from build123d import *

# Parameters (mm, degrees)
BOSS_EXTRUDE1_DEPTH = 13.85


with BuildPart() as part:
    # Sketch1 → Boss-Extrude1 (new, symmetric)
    with BuildSketch(Plane(origin=(0, 0, 0), x_dir=(0, 0, -1), z_dir=(1, 0, 0))):
        with BuildLine():
            ThreePointArc((75, 0), (-54.60082417, 51.417409503), (4.5, -74.864878281))
            Line((4.5, -74.864878281), (4.458, -74.166139417))
            ThreePointArc((4.458, -74.166139417), (-54.091216477, 50.937513681), (74.3, 0))
            ThreePointArc((74.3, 0), (66.712592514, -32.709631609), (45.5, -58.738743602))
            Line((45.5, -58.738743602), (45.5, -59.621724229))
            ThreePointArc((45.5, -59.621724229), (67.221648299, -33.260336739), (75, 0))
        make_face()
        with BuildLine():
            Line((4.458, -74.166139417), (4.5, -74.864878281))
            Line((4.5, -74.864878281), (4.5, -74.163602933))
            ThreePointArc((4.5, -74.163602933), (4.47900018, -74.164874148), (4.458, -74.166139417))
        make_face()
        with BuildLine():
            Line((45.075333333, -59.065254803), (45.5, -59.621724229))
            Line((45.5, -59.621724229), (45.5, -58.738743602))
            ThreePointArc((45.5, -58.738743602), (45.287960922, -58.902381917), (45.075333333, -59.065254803))
        make_face()
    extrude(amount=BOSS_EXTRUDE1_DEPTH, both=True)


solid = part.part
Verification items for the finished model (mm, model axes). Coordinates: 2 decimals unless noted, no trailing zeros. Loops run counter-clockwise (first coordinate to the right, second up) from the corner with the lowest first, then second, coordinate; pieces in that order, holes last. Notation, with made-up numbers: (82.25, 53.25) -> (112.25, 53.25) arc R21 ccw to (112.25, 57.25) -> close; hole circle Ø8 at (31.25, 16.5). An arc over 180 degrees is marked (long way). Answer as CSV lines item,"result".
1) Cross-section at D-D, the plane z = -38.5. Record the cut outline in (x, y).
Found:
outline,"(-13.85, 63.55) -> (13.85, 63.55) -> (13.85, 64.36) -> (-13.85, 64.36) -> close"
2) Cross-section at C-C, the plane x = 6.5. Record the cut outline in (y, z).
Found:
outline,"(-74.86, -4.5) -> (-74.16, -4.5) arc R74.3 cw to (-74.17, -4.46) arc R74.3 cw (long way) to (-58.74, -45.5) arc R74.3 cw to (-59.07, -45.08) -> (-59.62, -45.5) arc R75 ccw (long way) to start"
3) Cross-section at A-A, the plane z = 0. Record the cut outline in (x, y), then the cut area to 3 significant figures.
Found:
outline,"(-13.85, -75) -> (13.85, -75) -> (13.85, -74.3) -> (-13.85, -74.3) -> close; (-13.85, 74.3) -> (13.85, 74.3) -> (13.85, 75) -> (-13.85, 75) -> close"
area,"38.8 mm2"
4) Depth check by flat-ended pin: pin 1 (6 mm diameter, centred on x = -9, z = 50.5, fed in from -Y); pin 2 (1 mm diameter, centred on x = -7.5, y = -33, fed in from +Z); pin 3 (10 mm diameter, centred on x = -8, y = -50, fed in from -Z). Enter the tip coordinate at first touch or a pass-through.
Found:
pin 1,"stops at y = -58.04"
pin 2,"stops at z = 67.59"
pin 3,"stops at z = -60"
5) Thickness scan on L1, parallel to Y at x = 6.25, z = 0; L2, parallel to Y at x = -0.5, z = -57; L3, parallel to Z at x = 11.5, y = -21. Record the ranges inside material, lowest first. Write a range as from..to.
Found:
L1,"y = -75..-74.3, 74.3..75"
L2,"y = -48.74..-47.66, 47.66..48.74"
L3,"z = -72..-71.27, 71.27..72"
6) Cross-section at B-B, the plane y = 14.5. Record the cut outline in (x, z), then the cut area to 3 significant figures.
Found:
outline,"(-13.85, -73.58) -> (13.85, -73.58) -> (13.85, -72.87) -> (-13.85, -72.87) -> close; (-13.85, 72.87) -> (13.85, 72.87) -> (13.85, 73.58) -> (-13.85, 73.58) -> close"
area,"39.5 mm2"
7) Release check for a two-part mould opening along Y. For faces 1 (the flat face through (13.85, 17, 72.6)), 2 (the cylindrical face through (-0.194, 68.454, 28.889)) record: +Y half, -Y half, draft (parallel to the pull), parting line (faces both ways), or undercut.
Found:
face 1,"draft"
face 2,"undercut"
